Can you work these out from the drawing? Everything is in mm from the part's minimum corner. A direction names the side the tool comes from. Coordinates: 2 decimals unless noted, no trailing zeros. Loops run counter-clockwise (first coordinate to the right, second up) from the corner with the lowest first, then second, coordinate; pieces in that order, holes last.
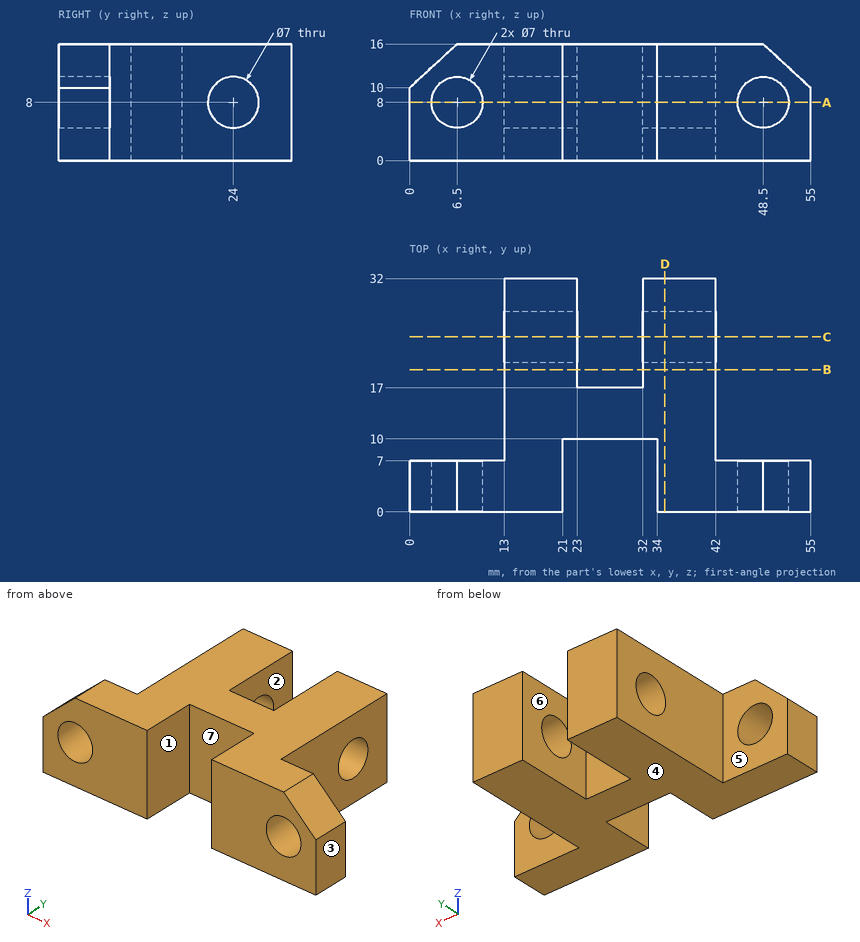
1) We'd pull the mould along X, two halves only. Please class the marked faces 1, 2, 3 and 4: released by +X, released by -X, zero draft, split by the parting line, or undercut.
2) Will these pins go through, and if not, where does the flat tip stop? pin 1 (4 mm diameter, centred on x = 30, z = 4.5, fed in from -Y); pin 2 (6 mm diameter, centred on y = 21, z = 13.5, fed in from -X); pin 3 (5 mm diameter, centred on x = 8, z = 9.5, fed in from +Y); pin 4 (8 mm diameter, centred on x = 10, z = 3.5, fed in from +Y).
3) Imagine slicing it at B-B on y = 19.5. List the corners of the cut face in (x, z) for me.
4) Imagine slicing it at A-A on z = 8. State how many separate pieces and enclosed holes the cut face has, plus the area to 3 significant figures.
5) Imagine slicing it at D-D on x = 35. List the corners of the cut face in (y, z) for me.
6) For the marked faces 5, 6 and 7, which set-ups out of +Z, -Z, +X, -X, +Y, -Y let a thin tool reach every point of the face, with its end or its side?
7) Imagine slicing it at C-C on y = 24. List the corners of the cut face in (x, z) for me, plus the area to 3 significant figures.
8) If I drill on L1, parallel to X at y = 4.25, z = 8; L2, parallel to X at y = 20, z = 13.5; L3, parallel to Z at x = 37.75, y = 24, over which ranges is the centre line in solid material (lowest first)?
Solved:
1. face 1: undercut
1. face 2: undercut
1. face 3: released by +X
1. face 4: zero draft
2. pin 1: stops at y = 10
2. pin 2: stops at x = 13
2. pin 3: stops at y = 7
2. pin 4: stops at y = 32
3. outline: (13, 0) - (23, 0) - (23, 16) - (13, 16) - close; (32, 0) - (42, 0) - (42, 16) - (32, 16) - close
4. separate pieces: 5
4. enclosed holes: 0
4. area: 607 mm2
5. outline: (0, 0) - (32, 0) - (32, 16) - (0, 16) - close; hole circle Ø7 at (24, 8)
6. face 5: +Z, -Z, -X, +Y
6. face 6: +Z, -Z, +Y
6. face 7: +Z, -Z, -Y
7. outline: (13, 0) - (23, 0) - (23, 4.5) - (13, 4.5) - close; (13, 11.5) - (23, 11.5) - (23, 16) - (13, 16) - close; (32, 0) - (42, 0) - (42, 4.5) - (32, 4.5) - close; (32, 11.5) - (42, 11.5) - (42, 16) - (32, 16) - close
7. area: 180 mm2
8. L1: x = 0 to 3, 10 to 21, 34 to 45, 52 to 55
8. L2: x = 13 to 23, 32 to 42
8. L3: z = 0 to 4.5, 11.5 to 16
